Work out the finished part from the listing and answer in its coordinate system (mm). Face numbers are marked on the shaded views. Round coordinates to 2 decimals unless told otherwise and drop trailing zeros. Write each loop counter-clockwise with the first axis right and the second up, starting at its lowest first coordinate (ties: lowest second). Pieces come first, ordered by that corner, then holes. Notation, with made-up numbers: (-5.75, -25.5) -> (2.25, -25.5) arc R11 cw to (2.25, -17.5) -> close; hole circle Ø2 at (80, 31.25). An arc over 180 degrees is marked (long way). Answer as a JSON object with one key per item and string values. Group by question number.
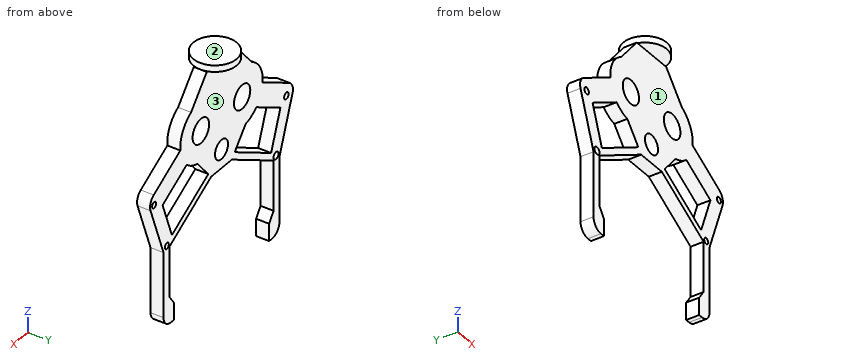
from build123d import *

# Parameters (mm, degrees)
SKETCH_1_R      = 5.517972707
SKETCH_1_R_2    = 5.611863705
SKETCH_1_R_3    = 1.527148593
SKETCH_1_R_4    = 1.382615372
SKETCH_1_R_5    = 1.672120879
SKETCH_1_R_6    = 1.371563178
SKETCH_1_R_7    = 4.42854447
EXTRUDE_1_DEPTH = 6
SKETCH_2_R      = 10
EXTRUDE_2_DEPTH = 3
FILLET_1_R      = 5


with BuildPart() as part:
    # 草图1 → 凸台-拉伸1 (new body)
    with BuildSketch(Plane(origin=(0, 0, 0), x_dir=(1, 0, 0), z_dir=(0, 1, 0))):
        with BuildLine():
            Line((-10, 0), (10, 0))
            Line((10, 0), (20.63165677, 12.67031515))
            ThreePointArc((20.63165677, 12.67031515), (26.297438403, 18.308736388), (27.95445115, 26.128402898))
            Line((27.95445115, 26.128402898), (49.605086245, 38.628402898))
            Line((49.605086245, 38.628402898), (39.344481945, 66.819181521))
            Line((39.344481945, 66.819181521), (39.344481945, 101.819181521))
            Line((39.344481945, 101.819181521), (32.344481945, 101.819181521))
            Line((32.344481945, 101.819181521), (32.344481945, 93.819181521))
            Line((32.344481945, 93.819181521), (35.344481945, 89.534737501))
            Line((35.344481945, 89.534737501), (35.344481945, 66.364694281))
            Line((35.344481945, 66.364694281), (7, 50))
            Line((7, 50), (-7, 50))
            Line((-7, 50), (-35.344481945, 66.364694281))
            Line((-35.344481945, 66.364694281), (-35.344481945, 89.534737501))
            Line((-35.344481945, 89.534737501), (-32.344481945, 93.819181521))
            Line((-32.344481945, 93.819181521), (-32.344481945, 101.819181521))
            Line((-32.344481945, 101.819181521), (-39.344481945, 101.819181521))
            Line((-39.344481945, 101.819181521), (-39.344481945, 66.819181521))
            Line((-39.344481945, 66.819181521), (-49.605086245, 38.628402898))
            Line((-49.605086245, 38.628402898), (-27.95445115, 26.128402898))
            ThreePointArc((-27.95445115, 26.128402898), (-26.297438403, 18.308736388), (-20.63165677, 12.67031515))
            Line((-20.63165677, 12.67031515), (-10, 0))
        make_face()
        with Locations(Location((-14, 25, 0), (0, 0, 270))):
            Circle(SKETCH_1_R, mode=Mode.SUBTRACT)
        with Locations(Location((14, 25, 0), (0, 0, 270))):
            Circle(SKETCH_1_R_2, mode=Mode.SUBTRACT)
        with Locations(Location((-44.044259413, 41.350104136, 0), (0, 0, 270))):
            Circle(SKETCH_1_R_3, mode=Mode.SUBTRACT)
        with Locations(Location((45.704626141, 41.350104136, 0), (0, 0, 270))):
            Circle(SKETCH_1_R_4, mode=Mode.SUBTRACT)
        with Locations(Location((-37.005131134, 65.009396406, 0), (0, 0, 270))):
            Circle(SKETCH_1_R_5, mode=Mode.SUBTRACT)
        with Locations(Location((37.145951464, 65.009396406, 0), (0, 0, 270))):
            Circle(SKETCH_1_R_6, mode=Mode.SUBTRACT)
        with Locations(Location((0, 41.350104136, 0), (0, 0, 270))):
            Circle(SKETCH_1_R_7, mode=Mode.SUBTRACT)
        with BuildLine():
            Line((8.958110934, 47.66641426), (16.404682223, 38.791936173))
            ThreePointArc((16.404682223, 38.791936173), (20.278324988, 37.51329834), (23.618950039, 35.172305548))
            Line((23.618950039, 35.172305548), (39.976426, 44.616298697))
            Line((39.976426, 44.616298697), (33.672776585, 61.935433126))
            Line((33.672776585, 61.935433126), (8.958110934, 47.66641426))
        make_face(mode=Mode.SUBTRACT)
        with BuildLine():
            Line((-8.958110934, 47.66641426), (-16.404682223, 38.791936173))
            ThreePointArc((-16.404682223, 38.791936173), (-20.278324988, 37.51329834), (-23.618950039, 35.172305548))
            Line((-23.618950039, 35.172305548), (-39.976426, 44.616298697))
            Line((-39.976426, 44.616298697), (-33.672776585, 61.935433126))
            Line((-33.672776585, 61.935433126), (-8.958110934, 47.66641426))
        make_face(mode=Mode.SUBTRACT)
    extrude(amount=EXTRUDE_1_DEPTH)

    # 草图2 → 凸台-拉伸2 (add)
    with BuildSketch(Plane.XY):
        with Locations((0, 3)):
            Circle(SKETCH_2_R)
    extrude(amount=EXTRUDE_2_DEPTH)

    # 圆角1
    fillet_1_edges = [part.edges().sort_by_distance(p)[0] for p in [
        (-49.605086245, 3, -38.628402898),
        (-39.344481945, 3, -101.819181521),
        (39.344481945, 3, -101.819181521),
        (49.605086245, 3, -38.628402898),
    ]]
    fillet(fillet_1_edges, radius=FILLET_1_R)


solid = part.part
1) A cutting plane is placed at A-A on x = 0. Determine the outline of the cut face in (y, z), plus the area to 3 significant figures.
2) A cutting plane is placed at C-C on x = -14. Determine the outline of the cut face in (y, z).
3) For a pull along Y with two mould halves and no side action, classify the marked faces 1, 2 and 3 as released by +Y, released by -Y, zero draft, split by the parting line, or undercut.
4) A cutting plane is placed at B-B on z = -71. Determine the outline of the cut face in (x, y).
5) A cutting plane is placed at D-D on y = 9. Determine the outline of the cut face in (x, z), plus the area to 3 significant figures.
6) Each of these flat-tipped pins is pushed along its axis until it touches: P1, Ø3, axis at y = 2.5, z = -80, coming from the -X side; P2, Ø3.5, axis at x = 45.7, z = -41.35, coming from the -Y side; P3, Ø10, axis at y = 5, z = -10.5, coming from the -X side. Where does it stop, or does it pass through?
7) Straight lines are drawn through the part: L1, parallel to X at y = 2.7, z = -25; L2, parallel to Z at x = -12.5, y = 3.75; L3, parallel to X at y = 5.5, z = -53 (3 decimals). For each, find the intervals that lie inside material, in ascending order.
Established:
{
 "1": {"outline": "(-7, 0) -> (0, 0) -> (0, -36.92) -> (6, -36.92) -> (6, 0) -> (13, 0) -> (13, 3) -> (-7, 3) -> close; (0, -50) -> (6, -50) -> (6, -45.78) -> (0, -45.78) -> close", "area": "307 mm²"},
 "2": {"outline": "(0, -54.04) -> (6, -54.04) -> (6, -50.58) -> (0, -50.58) -> close; (0, -41.66) -> (6, -41.66) -> (6, -30.52) -> (0, -30.52) -> close; (0, -19.48) -> (6, -19.48) -> (6, -4.77) -> (0, -4.77) -> close"},
 "3": {"face 1": "released by -Y", "face 2": "zero draft", "face 3": "released by +Y"},
 "4": {"outline": "(-39.34, 0) -> (-35.34, 0) -> (-35.34, 6) -> (-39.34, 6) -> close; (35.34, 0) -> (39.34, 0) -> (39.34, 6) -> (35.34, 6) -> close"},
 "5": {"outline": "(-8, 0) -> (8, 0) -> (8, 3) -> (-8, 3) -> close", "area": "48.0 mm²"},
 "6": {"P1": "stops at x = -39.34", "P2": "stops at y = 0", "P3": "stops at x = -24.28"},
 "7": {"L1": "x = -28 to -19.52, -8.48 to 8.39, 19.61 to 28", "L2": "z = -53.18 to -49.71, -43.45 to -30.31, -19.69 to -2.98", "L3": "x = -44.374 to -36.925, -18.196 to -12.196, 12.196 to 18.196, 36.925 to 44.374"}
}
